CAD build for the part. Positions are in the model's coordinates, mm. A direction names the side the tool comes from. Give positions to 0.01 mm unless a question says otherwise; leave off trailing zeros. Loops run counter-clockwise (first coordinate to the right, second up) from the corner with the lowest first, then second, coordinate; pieces in that order, holes last.
Item 1: Saw through at A-A on x = 0. Give the cut face in (y, z).
Item 2: Saw through at D-D on x = -34. Give the cut face in (y, z).
Item 3: Probe probe 1 along Y at (x, z) = (117, -1.5); probe 2 along X at (y, z) = (30, -8.5); probe 3 along Z at (x, y) = (49.5, 2). List the from-to ranges inside material, lowest first.
Item 4: Which spindle directions (+Z, -Z, +X, -X, +Y, -Y) get a long thin tool onto all of the face, cutting with end or side? Do faces 5 (the flat face through (22.5, -1, -28)), 6 (the flat face through (-10.3, 27.795, -43.5)), 7 (the cylindrical face through (147.59, 14.36, -12.4)). Say none if no direction does.
Item 5: Saw through at B-B on y = 0. Give the cut face in (x, z), plus the area to 3 significant figures.
Item 6: Saw through at C-C on x = 102. Give the cut face in (y, z).
Item 7: Mould opens along Y. For faces 1 (the flat face through (144.81, -50.16, -2.46)), 2 (the cylindrical face through (143.43, -17.18, -9.86)), 3 (the flat face through (-145, -14, -20)), 4 (the flat face through (145.29, 49.14, -2.46)) say: released by +Y, released by -Y, zero draft, split by the parting line, or undercut.
Item 8: Drop flat-ended pins along their axis: P1, Ø22.5, axis at x = 5, y = -7.5, coming from the -Z side; P2, Ø5, axis at x = 24.5, z = -32.5, coming from the -Y side; P3, Ø5.5, axis at x = -66, z = -1.5, coming from the -Y side. Give the stop position or say it passes through.
from build123d import *

# Parameters (mm, degrees)
SKETCH1_R           = 5
BOSS_EXTRUDE3_DEPTH = 5
BOSS_EXTRUDE4_DEPTH = 10
SKETCH1_6_R         = 47.8
SKETCH1_6_R_2       = 44.85
BOSS_EXTRUDE5_DEPTH = 20
SKETCH2_R           = 15
BOSS_EXTRUDE6_DEPTH = 88
SKETCH3_W           = 90.131554877
SKETCH3_H           = 60.595357862
CUT_EXTRUDE1_DEPTH  = 57


with BuildPart() as part:
    # Sketch1 → Boss-Extrude3 (new body)
    with BuildSketch(Plane.XY):
        Polygon((-18, 86), (-128.1, 86), (-162, 13.3), (-162, -13.3), (-128.1, -86), (-18, -86), (-18, -95), (18, -95), (18, -86), (128.1, -86), (162, -13.3), (162, 13.3), (128.1, 86), (18, 86), (18, 95), (-18, 95), align=None)
        with Locations((-117, -73.410936815)):
            Circle(SKETCH1_R, mode=Mode.SUBTRACT)
        with Locations((117, -73.410936815)):
            Circle(SKETCH1_R, mode=Mode.SUBTRACT)
        with BuildLine():
            ThreePointArc((-83.3227411, -44), (-149.8, 0), (-83.3227411, 44))
            Line((-83.3227411, 44), (83.3227411, 44))
            ThreePointArc((83.3227411, 44), (128.382447049, 39.85983552), (149.8, 0))
            ThreePointArc((149.8, 0), (128.382447049, -39.85983552), (83.3227411, -44))
            Line((83.3227411, -44), (-83.3227411, -44))
        make_face(mode=Mode.SUBTRACT)
        with Locations((-117, 73.410936815)):
            Circle(SKETCH1_R, mode=Mode.SUBTRACT)
        with Locations((117, 73.410936815)):
            Circle(SKETCH1_R, mode=Mode.SUBTRACT)
    extrude(amount=-BOSS_EXTRUDE3_DEPTH)

    # Sketch1<5> → Boss-Extrude4 (add)
    with BuildSketch(Plane.XY):
        with BuildLine():
            Line((83.3227411, 44), (-83.3227411, 44))
            ThreePointArc((-83.3227411, 44), (-62.14016448, 26.382447049), (-54.2, 0))
            ThreePointArc((-54.2, 0), (-62.14016448, -26.382447049), (-83.3227411, -44))
            Line((-83.3227411, -44), (83.3227411, -44))
            ThreePointArc((83.3227411, -44), (54.2, 0), (83.3227411, 44))
        make_face()
    extrude(amount=-BOSS_EXTRUDE4_DEPTH)

    # Sketch1<6> → Boss-Extrude5 (add)
    # profile 1 of 2: a face of its own
    with BuildSketch(Plane.XY):
        with Locations((102, 0)):
            Circle(SKETCH1_6_R)
        with Locations((102, 0)):
            Circle(SKETCH1_6_R_2, mode=Mode.SUBTRACT)
    # profile 2 of 2: a face of its own
    with BuildSketch(Plane.XY):
        with Locations((-102, 0)):
            Circle(SKETCH1_6_R)
        with Locations((-102, 0)):
            Circle(SKETCH1_6_R_2, mode=Mode.SUBTRACT)
    extrude(amount=-BOSS_EXTRUDE5_DEPTH)

    # Sketch2 → Boss-Extrude6 (add)
    with BuildSketch(Plane.XZ.offset(44)):
        with BuildLine():
            Line((22.5, -55), (22.5, -10))
            Line((22.5, -10), (-22.5, -10))
            Line((-22.5, -10), (-22.5, -55))
            ThreePointArc((-22.5, -55), (0, -77.5), (22.5, -55))
        make_face()
        with Locations((0, -55)):
            Circle(SKETCH2_R, mode=Mode.SUBTRACT)
    extrude(amount=-BOSS_EXTRUDE6_DEPTH)

    # Sketch3 → Cut-Extrude1 (cut)
    with BuildSketch(Plane.ZY.offset(22.5)):
        with Locations((-75.065777439, -2.502321069)):
            Rectangle(SKETCH3_W, SKETCH3_H)
    extrude(amount=-CUT_EXTRUDE1_DEPTH, mode=Mode.SUBTRACT)


solid = part.part
Results below:
1. outline: (-95, -5) - (-44, -5) - (-44, -40) - (-32.8, -40) - (-32.8, -30) - (27.8, -30) - (27.8, -40) - (44, -40) - (44, -5) - (95, -5) - (95, 0) - (-95, 0) - close; (-44, -77.5) - (-32.8, -77.5) - (-32.8, -70) - (-44, -70) - close; (27.8, -77.5) - (44, -77.5) - (44, -70) - (27.8, -70) - close
2. outline: (-86, -5) - (-44, -5) - (-44, -10) - (44, -10) - (44, -5) - (86, -5) - (86, 0) - (-86, 0) - close
3. probe 1: y = -86 to -78.41, -68.41 to -42.27, 42.27 to 68.41, 78.41 to 86
3. probe 2: x = -139.21 to -135.34, -68.66 to 68.66, 135.34 to 139.21
3. probe 3: z = -10 to 0
4. face 5: -Z, +Y, -Y
4. face 6: -Z, +X, -X
4. face 7: -Z
5. outline: (-162, -5) - (-149.8, -5) - (-149.8, -20) - (-146.85, -20) - (-146.85, 0) - (-162, 0) - close; (-57.15, -20) - (-54.2, -20) - (-54.2, -10) - (-22.5, -10) - (-22.5, -30) - (22.5, -30) - (22.5, -10) - (54.2, -10) - (54.2, -20) - (57.15, -20) - (57.15, 0) - (-57.15, 0) - close; (146.85, -20) - (149.8, -20) - (149.8, -5) - (162, -5) - (162, 0) - (146.85, 0) - close
5. area: 2,340 mm2
6. outline: (-86, -5) - (-47.8, -5) - (-47.8, -20) - (-44.85, -20) - (-44.85, 0) - (-86, 0) - close; (44.85, -20) - (47.8, -20) - (47.8, -5) - (86, -5) - (86, 0) - (44.85, 0) - close
7. face 1: released by -Y
7. face 2: undercut
7. face 3: zero draft
7. face 4: released by +Y
8. P1: stops at z = -30
8. P2: stops at y = -44
8. P3: stops at y = -86
